Source: CAD feature listing. Evaluate the final solid. Frame: model axes, mm. Give positions to 0.01 mm unless a question says otherwise; leave off trailing zeros. Write each loop counter-clockwise with the first axis right and the second up, starting at its lowest first coordinate (ties: lowest second). Pieces come first, ordered by that corner, then holes. Notation, with made-up numbers: M -10.75,55 L -2.75,55 A18 ccw -2.75,70 Z; hole C 33.25,63 d1. An arc over 180 degrees is marked long. Return JSON: item names as keys, results as strings.
```python
from build123d import *

# Parameters (mm, degrees)
BASE_FLANGE1_DEPTH       = 612.775
CUT_EXTRUDE1_OUTLINE_W   = 38.1
CUT_EXTRUDE1_OUTLINE_H   = 57.651763494
CUT_EXTRUDE1_DEPTH       = 33.236308369
CUT_EXTRUDE1_START       = -3.175
CUT_EXTRUDE1_2_OUTLINE_W = 38.1
CUT_EXTRUDE1_2_OUTLINE_H = 6.35
CUT_EXTRUDE1_2_DEPTH     = 3.175
SKETCH7_R                = 4.3688
CUT_EXTRUDE2_DEPTH       = 3.175
SKETCH8_R                = 3.429
CUT_EXTRUDE3_DEPTH       = 3.175
FILLET1_R                = 3.175


# Read off the part's stored shape, not the designer's step: Cut-Extrude1
# Sheet-metal steps are written as plain solids
with BuildPart() as part:
    # Sketch1 → Base-Flange1 (new body)
    with BuildSketch(Plane(origin=(0, 0, 0), x_dir=(0, 0, -1), z_dir=(1, 0, 0))):
        with BuildLine():
            Line((0, 0), (0, 51.301763494))
            ThreePointArc((0, 51.301763494), (3.417896306, 56.934282284), (9.992210371, 56.503378975))
            Line((9.992210371, 56.503378975), (36.411308369, 38.004527404))
            Line((36.411308369, 38.004527404), (34.590203183, 35.403719664))
            Line((34.590203183, 35.403719664), (8.171105185, 53.902571234))
            ThreePointArc((8.171105185, 53.902571234), (4.883948153, 54.118022889), (3.175, 51.301763494))
            Line((3.175, 51.301763494), (3.175, 0))
            Line((3.175, 0), (0, 0))
        make_face()
    extrude(amount=BASE_FLANGE1_DEPTH)

    # Cut-Extrude1 outline → Cut-Extrude1 (cut)
    with BuildSketch(Plane(origin=(0, 0, -3.175), x_dir=(-1, 0, 0), z_dir=(0, 0, -1))):
        with Locations((-593.725, 28.825881747)):
            Rectangle(CUT_EXTRUDE1_OUTLINE_W, CUT_EXTRUDE1_OUTLINE_H)
        with Locations((-19.05, 28.825881747)):
            Rectangle(CUT_EXTRUDE1_OUTLINE_W, CUT_EXTRUDE1_OUTLINE_H)
    extrude(amount=CUT_EXTRUDE1_DEPTH, mode=Mode.SUBTRACT)

    # Cut-Extrude1 2 outline → Cut-Extrude1 2 (cut)
    with BuildSketch(Plane(origin=(0, 0, -3.175), x_dir=(-1, 0, 0), z_dir=(0, 0, -1)).offset(CUT_EXTRUDE1_START)):
        with Locations((-593.725, 54.476763494)):
            Rectangle(CUT_EXTRUDE1_2_OUTLINE_W, CUT_EXTRUDE1_2_OUTLINE_H)
        with Locations((-19.05, 54.476763494)):
            Rectangle(CUT_EXTRUDE1_2_OUTLINE_W, CUT_EXTRUDE1_2_OUTLINE_H)
    extrude(amount=CUT_EXTRUDE1_2_DEPTH, mode=Mode.SUBTRACT)

    # Sketch7 → Cut-Extrude2 (cut)
    with BuildSketch(Plane.XY):
        with Locations((15.875, 39.109763494)):
            Circle(SKETCH7_R)
        with Locations((15.875, 20.059763494)):
            Circle(SKETCH7_R)
        with Locations((596.9, 39.109763494)):
            Circle(SKETCH7_R)
        with Locations((596.9, 20.059763494)):
            Circle(SKETCH7_R)
    extrude(amount=-CUT_EXTRUDE2_DEPTH, mode=Mode.SUBTRACT)

    # Sketch8 → Cut-Extrude3 (cut)
    with BuildSketch(Plane(origin=(0, 42.609139551, -29.83524071), x_dir=(1, 0, 0), z_dir=(0, 0.819152044288989, -0.5735764363510502))):
        with Locations(Location((560.3875, 0.090396292, 0), (0, 0, 270))):
            Circle(SKETCH8_R)
        with Locations(Location((52.3875, 0.090396292, 0), (0, 0, 270))):
            Circle(SKETCH8_R)
    extrude(amount=-CUT_EXTRUDE3_DEPTH, mode=Mode.SUBTRACT)

    # Fillet1
    fillet1_edges = [part.edges().sort_by_distance(p)[0] for p in [
        (0, 51.301763494, -1.5875),
        (612.775, 51.301763494, -1.5875),
        (612.775, 0, -1.5875),
        (38.1, 36.704123534, -35.500755776),
        (574.675, 36.704123534, -35.500755776),
        (0, 0, -1.5875),
    ]]
    fillet(fillet1_edges, radius=FILLET1_R)


solid = part.part
```
1) Line query: line 1 (Z direction, x = 552, y = 20) (3 decimals); line 2 (Z direction, x = 556, y = 43.5) (3 decimals); line 3 (Z direction, x = 67, y = 53). Output: solid intervals per line, ascending. Write a range as [from, to].
Numbers:
{"line 1": "z = [-3.175, 0]", "line 2": "z = [-28.563, -23.028], [-3.175, 0]", "line 3": "z = [-15, -9.46], [-3.67, -0.23]"}
2) Cut plane A-A, the plane x = 435. Return the cut outline in (y, z) (3 decimals).
Numbers:
{"outline": "M 0,-3.175 L 51.302,-3.175 A3.175 cw 53.903,-8.171 L 35.404,-34.59 L 38.005,-36.411 L 56.503,-9.992 A6.35 ccw 51.302,0 L 0,0 Z"}
3) Contact query for flat-ended pins moving along their axis: pin 1 Ø1.5 at (y, z) = (39.5, -25) entering from +X; pin 2 Ø11.5 at (x, y) = (15.88, 39.11) entering from -Z (3 decimals); pin 3 Ø1.6 at (x, z) = (29, -1) entering from +Y; pin 4 Ø16.5 at (y, z) = (48.5, -11.5) entering from -X. Output: stop coordinate, or through.
Numbers:
{"pin 1": "passes through", "pin 2": "stops at z = -3.175", "pin 3": "stops at y = 51.3", "pin 4": "stops at x = 38.1"}
4) Draft query along Z for faces 1 (the face through (302, 25, 0)), 2 (the face through (302.6, 44.5, -21.6)), 3 (the face through (302.63, 47.38, -23.02)), 4 (the face through (302, 26, -3.175)). Return one class per face: released by +Z, released by -Z, zero draft, split by the parting line, or undercut.
Numbers:
{"face 1": "released by +Z", "face 2": "undercut", "face 3": "released by -Z", "face 4": "undercut"}
